Here's how the part is built. I have some questions about the finished solid (model axes, mm). A direction names the side the tool comes from. Round coordinates to 2 decimals unless told otherwise and drop trailing zeros. Order: outer loops, then holes, each group sorted by start corner. A loop starts at its lowest first (then second) coordinate and runs counter-clockwise, first axis right, second up. Notation, with made-up numbers: (22.5, -6.75) -> (48.5, -6.75) arc R32 cw to (48.5, 19.25) -> close; hole circle Ø11 at (74.25, 49.25). An arc over 180 degrees is marked (long way). One line per item, written item: value.
Autodesk Fusion 360 part; units mm, degrees
sketch "Sketch1" plane through (0, 0, 0) normal (0, 0, 1) x (1, 0, 0)
  line L0 (0, 0) -> (100, 0)
  line L1 (0, 0) -> (0, 50)
  line L2 (0, 50) -> (30, 50)
  line L3 (30, 50) -> (30, 40)
  line L4 (60, 40) -> (60, 30)
  line L5 (60, 30) -> (100, 30)
  line L6 (100, 30) -> (100, 0)
  line L7 (50, 40) -> (50, 36)
  line L8 (50, 36) -> (42, 36)
  line L9 (42, 36) -> (42, 40)
  line L10 (30, 40) -> (42, 40)
  line L11 (50, 40) -> (60, 40)
  dimension "d1" = 100
  dimension "d2" = 50
  dimension "d3" = 4
  dimension "d4" = 8
revolve "Revolve1" add sketch "Sketch1" angle 360 about axis through (0, 0, 0) along (1, 0, 0)
sketch "Sketch2" plane through (100, 0, 0) normal (1, 0, 0) x (0, 1, 0)
  circle A0 centre (0, 0) radius 30
hole "Hole1" at (100, 0, 0) direction (-1, 0, 0) diameter 16 end through all
Q1. I want a section at A-A on z = 0. Write out the boundary of the cut face in (x, y), then the cut area to 3 significant figures.
Answers:
outline: (0, -50) -> (30, -50) -> (30, -40) -> (42, -40) -> (42, -36) -> (50, -36) -> (50, -40) -> (60, -40) -> (60, -30) -> (100, -30) -> (100, -8) -> (0, -8) -> close; (0, 8) -> (100, 8) -> (100, 30) -> (60, 30) -> (60, 40) -> (50, 40) -> (50, 36) -> (42, 36) -> (42, 40) -> (30, 40) -> (30, 50) -> (0, 50) -> close
area: 6,140 mm2
Q2. I need wall thicknesses on line 1 along Z through (x, y) = (21, 0); line 2 along Z through (x, y) = (32.5, 0); line 3 along X through (y, z) = (-31.5, -30). Which ranges of each line are inside material? Lowest first, please.
Answers:
line 1: -50 to -8, 8 to 50
line 2: -40 to -8, 8 to 40
line 3: 0 to 30
Q3. For P1, Ø10, axis at y = 1.5, z = 34, coming from the +X side; P2, Ø4, axis at x = 41.5, y = -29, coming from the +Z side; P3, Ø1, axis at x = 87.5, z = 7.5, coming from the -Y side; P4, Ø1.5, axis at x = 43.5, z = 25, coming from the +Y side, each with a flat end and sliding along its axis, tell me the tip position at first contact or that it passes through.
Answers:
P1: x = 100
P2: z = 29.51
P3: y = -29.17
P4: y = 26.61
Q4. If we mould it in two halves opening along Y, with no side actions, what happens to faces 4 (the face through (30, -22, 34)), 5 (the face through (80.28, -29.97, 1.32)), 6 (the face through (49.3, 7.81, 1.73))? For each: pulls with the +Y half, pulls with the -Y half, needs draft (parallel to the pull), parting line crosses it, or undercut.
Answers:
face 4: needs draft
face 5: parting line crosses it
face 6: undercut
Q5. I want a section at D-D on y = -16. Write out the boundary of the cut face in (x, z), then the cut area to 3 significant figures.
Answers:
outline: (0, -47.37) -> (30, -47.37) -> (30, -36.66) -> (42, -36.66) -> (42, -32.25) -> (50, -32.25) -> (50, -36.66) -> (60, -36.66) -> (60, -25.38) -> (100, -25.38) -> (100, 25.38) -> (60, 25.38) -> (60, 36.66) -> (50, 36.66) -> (50, 32.25) -> (42, 32.25) -> (42, 36.66) -> (30, 36.66) -> (30, 47.37) -> (0, 47.37) -> close
area: 7,000 mm2
Q6. Which directions (+Z, -Z, +X, -X, +Y, -Y) give clear straight access to the entire face, cutting with the end or side of a thin tool? Please do faces 1 (the face through (45.944, -4.686, -35.694)), 2 (the face through (36.08, -8.67, -39.05)), 3 (the face through (0, -1, -10)).
Answers:
face 1: none
face 2: +X
face 3: +Z, -Z, -X, +Y, -Y
Q7. I want a section at C-C on x = 14. Write out the boundary of the cut face in (y, z), then the cut area to 3 significant figures.
Answers:
outline: circle Ø100 at (0, 0); hole circle Ø16 at (0, 0)
area: 7,650 mm2
